Check sheet for the modelled part. Datum: model origin and axes. Units: mm. Give positions to 0.01 mm unless a question says otherwise; leave off trailing zeros. Order: outer loops, then holes, each group sorted by start corner. A loop starts at its lowest first (then second) coordinate and runs counter-clockwise, first axis right, second up.
from build123d import *

# Parameters (mm, degrees)
SKETCH1_R                  = 95.25
F001_EXTRUDE_BOSS_DEPTH    = 12.7
SKETCH2_R                  = 49.276
F002_HOLE_DEPTH            = 270.706859386
SKETCH3_R                  = 5.1562
F003_SEEDHOLECUT_DEPTH     = 270.706859386
F003_CIRCULARPATTERN_COUNT = 6
SKETCH4_R                  = 15.875
F004_EXTRUDE_CUT_DEPTH     = 270.706859386


with BuildPart() as part:
    # Sketch1 → F001_extrude_boss (new body)
    with BuildSketch(Plane.XY):
        with Locations((95.25, 95.25)):
            Circle(SKETCH1_R)
    extrude(amount=F001_EXTRUDE_BOSS_DEPTH)

    # Sketch2 → F002_hole (cut, through all)
    with BuildSketch(Plane.XY):
        with Locations((95.25, 95.25)):
            Circle(SKETCH2_R)
    extrude(amount=F002_HOLE_DEPTH, mode=Mode.SUBTRACT)

    # Sketch3 → F003_SeedHoleCut (cut, through all)
    with BuildSketch(Plane.XY):
        with Locations((58.6751176, 31.900445402)):
            Circle(SKETCH3_R)
    f003_seedholecut = extrude(amount=F003_SEEDHOLECUT_DEPTH, mode=Mode.SUBTRACT)

    # F003_CircularPattern: F003_SeedHoleCut ×6 about axis
    f003_circularpattern_axis = Axis((95.25, 95.25, 0), (0, 0, 1))
    for i in range(1, F003_CIRCULARPATTERN_COUNT):
        add(f003_seedholecut.rotate(f003_circularpattern_axis, i * 360 / F003_CIRCULARPATTERN_COUNT), mode=Mode.SUBTRACT)

    # Sketch4 → F004_extrude_cut (cut, through all)
    with BuildSketch(Plane.XY):
        with Locations((95.25, 20.574)):
            Circle(SKETCH4_R)
    extrude(amount=F004_EXTRUDE_CUT_DEPTH, mode=Mode.SUBTRACT)


solid = part.part
1) Depth check by flat-ended pin: pin 1 Ø1 at (y, z) = (127.5, 4.5) entering from +X; pin 2 Ø4 at (y, z) = (88.5, 3.5) entering from +X; pin 3 Ø2 at (y, z) = (171, 2) entering from +X. Enter the tip coordinate at first touch or a pass-through.
Recorded:
pin 1: stops at x = 185.05
pin 2: stops at x = 190.38
pin 3: stops at x = 154.28
2) Section check C-C, the plane x = 71. Record the cut outline in (y, z), then the cut area to 3 significant figures.
Recorded:
outline: (3.14, 0) - (52.35, 0) - (52.35, 12.7) - (3.14, 12.7) - close; (138.15, 0) - (187.36, 0) - (187.36, 12.7) - (138.15, 12.7) - close
area: 1,250 mm2
3) Section check A-A, the plane y = 95.25. Record the cut outline in (x, z).
Recorded:
outline: (0, 0) - (16.94, 0) - (16.94, 12.7) - (0, 12.7) - close; (27.26, 0) - (45.97, 0) - (45.97, 12.7) - (27.26, 12.7) - close; (144.53, 0) - (163.24, 0) - (163.24, 12.7) - (144.53, 12.7) - close; (173.56, 0) - (190.5, 0) - (190.5, 12.7) - (173.56, 12.7) - close
4) Section check D-D, the plane z = 9. State how many separate pieces and enclosed holes the cut face has, then the cut area to 3 significant figures.
Recorded:
separate pieces: 1
enclosed holes: 8
area: 19,600 mm2
5) Draft check along X on faces 1 (the face through (25.047, 159.624, 6.261)), 2 (the face through (58, 163.71, 6.26)), 3 (the face through (136, 54, 0)). Enter one of: +X half, -X half, draft (parallel to the pull), parting line (faces both ways), or undercut.
Recorded:
face 1: parting line
face 2: undercut
face 3: draft
6) Material ranges on L1, parallel to Y at x = 95.25, z = 8.25; L2, parallel to X at y = 96.5, z = 3.75; L3, parallel to X at y = 34.5, z = 5, recorded low to high.
Recorded:
L1: y = 0 to 4.7, 36.45 to 45.97, 144.53 to 190.5
L2: x = 0.01 to 17.1, 27.1 to 45.99, 144.51 to 163.4, 173.4 to 190.49
L3: x = 21.89 to 54.22, 63.13 to 87.63, 102.87 to 127.37, 136.28 to 168.61
7) Section check B-B, the plane x = 95.25. Record the cut outline in (y, z).
Recorded:
outline: (0, 0) - (4.7, 0) - (4.7, 12.7) - (0, 12.7) - close; (36.45, 0) - (45.97, 0) - (45.97, 12.7) - (36.45, 12.7) - close; (144.53, 0) - (190.5, 0) - (190.5, 12.7) - (144.53, 12.7) - close
